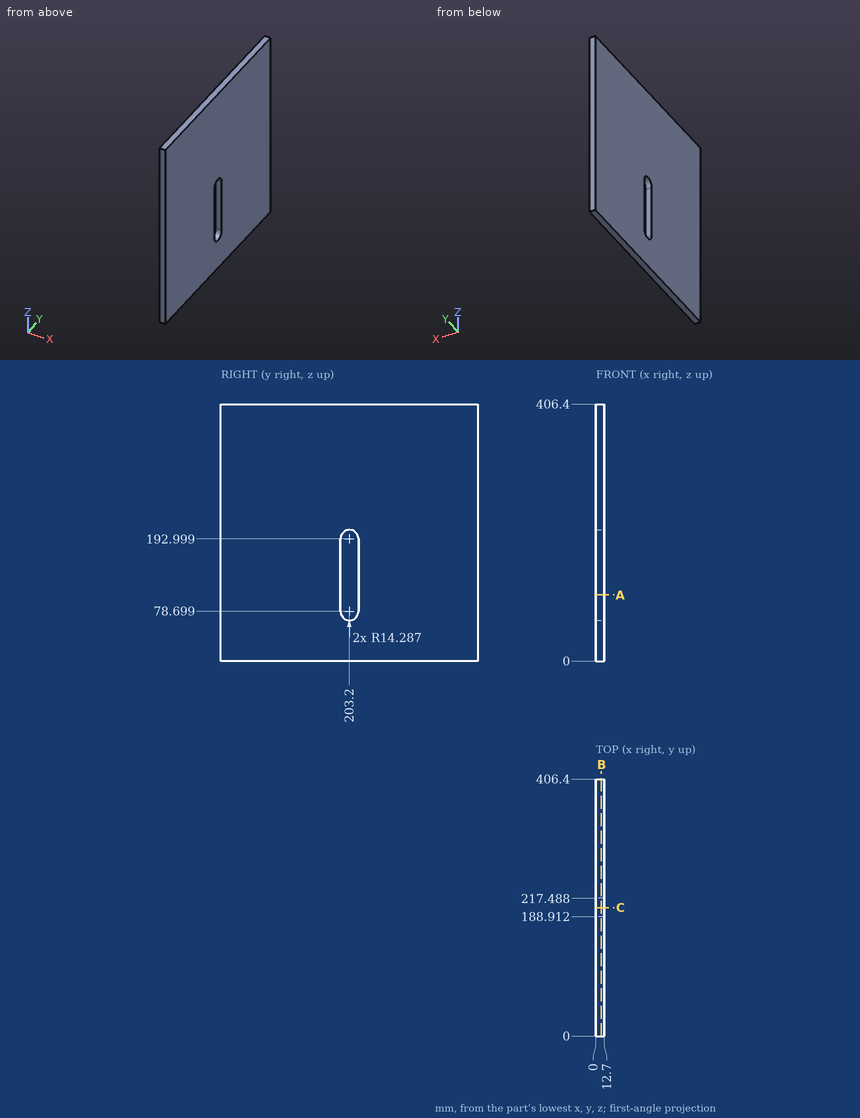
Can you work these out from the drawing? Everything is in mm from the part's minimum corner. Give positions to 0.01 mm unless a question says otherwise; leave off trailing zeros. Order: outer loops, then holes, each group sorted by start corner. A loop starts at its lowest first (then second) coordinate and runs counter-clockwise, first axis right, second up. Notation, with made-up numbers: M 40,-25 L 65,-25 A20 cw 65,-7 Z; hole C 87.25,43 d1. An arc over 180 degrees is marked long. One line per question, with ' | ' between items.
1. I want a section at A-A (z = 104.5). List the corners of the cut face in (x, y) for me, and give its area (3 significant figures).
Results:
outline: M 0,0 L 12.7,0 L 12.7,188.91 L 0,188.91 Z; M 0,217.49 L 12.7,217.49 L 12.7,406.4 L 0,406.4 Z | area: 4,800 mm²
2. I want a section at C-C (y = 203.2). List the corners of the cut face in (x, z) for me.
Results:
outline: M 0,0 L 12.7,0 L 12.7,64.41 L 0,64.41 Z; M 0,207.29 L 12.7,207.29 L 12.7,406.4 L 0,406.4 Z
3. If I drill on line 1 (Y direction, x = 5, z = 121); line 2 (Y direction, x = 7.75, z = 198) (1 decimal), over which ranges is the centre line in solid material (lowest first)?
Results:
line 1: 0 to 188.91, 217.49 to 406.4 | line 2: 0 to 189.8, 216.6 to 406.4
4. I want a section at B-B (x = 8.5). List the corners of the cut face in (y, z) for me (1 decimal), and give its area (3 significant figures).
Results:
outline: M 0,0 L 406.4,0 L 406.4,406.4 L 0,406.4 Z; hole M 188.9,78.7 A14.3 ccw 217.5,78.7 L 217.5,193 A14.3 ccw 188.9,193 Z | area: 161,000 mm²
